For this review, use the dimensioned drawing (mm, ordinates from the lowest corner) and the shaded views. A direction names the side the tool comes from. Give positions to 0.01 mm unless a question says otherwise; leave off trailing zeros. Loops run counter-clockwise (first coordinate to the right, second up) from the corner with the lowest first, then second, coordinate; pieces in that order, holes last. Notation, with made-up numbers: M -36.75,-5.75 L -23.75,-5.75 A11 cw -23.75,-1.75 Z; hole C -18,54.5 d4. An arc over 180 degrees is marked long. Use CSV: the item, a comma, the result in double quotes. Start each with the question number.
1. Tool access review of the marked faces 4, 5, 6 and 7: name each direction out of +Z, -Z, +X, -X, +Y, -Y from which nothing blocks a thin tool from reaching the whole face with its end or side.
2. Take a section at D-D, the plane z = 40.5. Write out the cut boundary in (x, y).
3. Take a section at B-B, the plane x = 41. Write out the cut boundary in (y, z).
4. The part is to be moulded in two halves that separate along Z. For the marked faces 1, 2 and 3, say which applies: pulls with the +Z half, pulls with the -Z half, needs draft (parallel to the pull), parting line crosses it, or undercut.
5. Insertion check: P1, Ø4, axis at y = 31, z = 11, coming from the +X side; P2, Ø10, axis at y = 18, z = 4.5, coming from the -X side; P3, Ø1.5, axis at y = 8.5, z = 54, coming from the -X side (1 decimal). Each pin has a flat end and moves straight along its axis. Give the tip position at first contact, or say it passes through.
6. To check wall thickness, follow line 1 (Z direction, x = 63, y = 12) (1 decimal); line 2 (Z direction, x = 63.5, y = 48.75); line 3 (X direction, y = 5, z = 7). State the ranges of each line that lie inside material, in increasing order. Write a range as [from, to].
7. Take a section at C-C, the plane x = 8.5. Write out the cut boundary in (y, z).
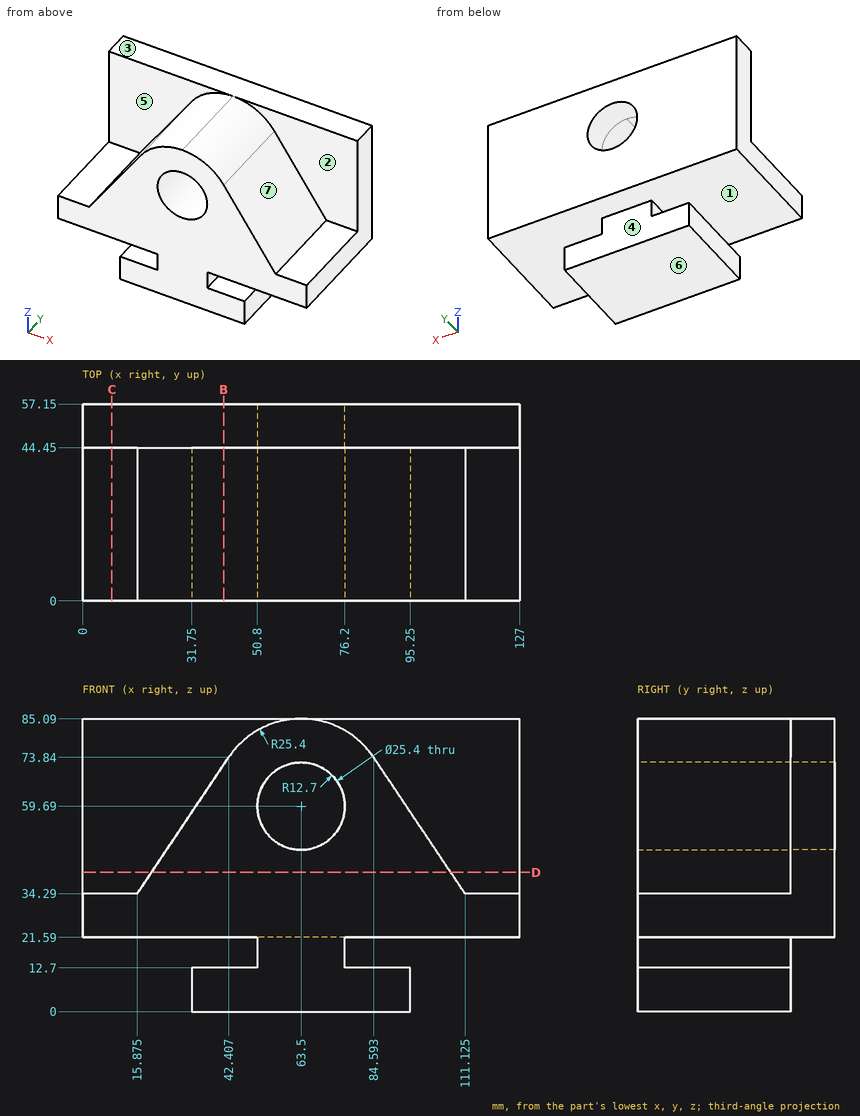
Result set:
1,face 4,"-Z, +X, -X, +Y"
1,face 5,"+Z, -X, -Y"
1,face 6,"-Z, +X, -X, +Y, -Y"
1,face 7,"+Z, +X, -Y"
2,outline,"M 0,44.45 L 20.04,44.45 L 20.04,0 L 106.96,0 L 106.96,44.45 L 127,44.45 L 127,57.15 L 0,57.15 Z"
3,outline,"M 0,0 L 44.45,0 L 44.45,12.7 L 0,12.7 Z; M 0,21.59 L 57.15,21.59 L 57.15,85.09 L 44.45,85.09 L 44.45,71.74 L 0,71.74 Z"
4,face 1,"undercut"
4,face 2,"needs draft"
4,face 3,"pulls with the +Z half"
5,P1,"x = 95.25"
5,P2,"x = 31.75"
5,P3,"x = 28.6"
6,line 1,"[0, 47], [72.4, 85.1]"
6,line 2,"[21.59, 46.99], [72.39, 85.09]"
6,line 3,"[31.75, 95.25]"
7,outline,"M 0,21.59 L 57.15,21.59 L 57.15,85.09 L 44.45,85.09 L 44.45,34.29 L 0,34.29 Z"
